Here's how the part is built. I have some questions about the finished solid (model axes, mm). A direction names the side the tool comes from. Round coordinates to 2 decimals unless told otherwise and drop trailing zeros. Order: outer loops, then holes, each group sorted by start corner. A loop starts at its lowest first (then second) coordinate and runs counter-clockwise, first axis right, second up. Notation, with made-up numbers: (78.5, 36.25) -> (130.5, 36.25) arc R27 ccw to (130.5, 69.25) -> close; hole circle Ø3 at (21.5, 54). An arc over 180 degrees is marked (long way). Answer in a Markdown table with one row per item.
```python
from build123d import *

# Parameters (mm, degrees)
F1_DEPTH  = 14
F3_W      = 7
F3_H      = 3.5
F4_DEPTH  = 16
F5_W      = 5
F5_H      = 0.4111507442
F5_H_2    = 17
F6_DEPTH  = 1.9
F8_R      = 0.99999
F10_DEPTH = 1.5
F11_W     = 2.5
F11_H     = 18.2
F12_DEPTH = 4.2
F13_W     = 2.5
F13_H     = 18.2
F14_DEPTH = 1.35
F15_W     = 3
F15_H     = 3
F16_DEPTH = 0.1
F17_DEPTH = 15
F18_R     = 5
F19_W     = 2.0917450339
F19_H     = 2.5
F20_DEPTH = 28.001
F19_W_2   = 2.772427164
F21_DEPTH = 28.001


# Not quite as in the source:
# - a fillet or chamfer is up to 0.001 mm smaller than in the source, because OpenCascade refuses the exact size
# - the program builds the solid bodies; features that only make, move or delete a surface that nothing else refers to are left out


with BuildPart() as f1:
    # F0 (on Front) → F1 (new body, symmetric)
    with BuildSketch(Plane.XZ):
        with BuildLine():
            Line((10, -6), (14, -6))
            Line((14, -6), (14, 6))
            Line((14, 6), (-14, 6))
            Line((-14, 6), (-14, -6))
            Line((-14, -6), (-10, -6))
            Line((-10, -6), (-4.7058823529, -3.1764705882))
            ThreePointArc((-4.7058823529, -3.1764705882), (0, -2), (4.7058823529, -3.1764705882))
            Line((4.7058823529, -3.1764705882), (10, -6))
        make_face()
        with BuildLine():
            Line((-10, -6), (10, -6))
            Line((10, -6), (4.7058823529, -3.1764705882))
            ThreePointArc((4.7058823529, -3.1764705882), (0, -2), (-4.7058823529, -3.1764705882))
            Line((-4.7058823529, -3.1764705882), (-10, -6))
        make_face()
    extrude(amount=F1_DEPTH, both=True)

    # F3 (on face) → F4 (cut)
    with BuildSketch(Plane.XZ.offset(14)):
        with Locations((0, 4.25)):
            Rectangle(F3_W, F3_H)
    extrude(amount=-F4_DEPTH, mode=Mode.SUBTRACT)

    # F5 (on face) → F6 (join)
    with BuildSketch(Plane.XY.offset(6)):
        with BuildLine():
            Line((2.5, -15), (-2.5, -15))
            Line((-2.5, -15), (-4, -15))
            ThreePointArc((-4, -15), (-5.4142135624, -15.5857864376), (-6, -17))
            Line((-6, -17), (-6, -18.5))
            ThreePointArc((-6, -18.5), (-5.267766953, -20.267766953), (-3.5, -21))
            Line((-3.5, -21), (3.5, -21))
            ThreePointArc((3.5, -21), (5.267766953, -20.267766953), (6, -18.5))
            Line((6, -18.5), (6, -17))
            ThreePointArc((6, -17), (5.4142135624, -15.5857864376), (4, -15))
            Line((4, -15), (2.5, -15))
        make_face()
        with Locations((0, 2.2055753721)):
            Rectangle(F5_W, F5_H)
        with Locations((0, -6.5)):
            Rectangle(F5_W, F5_H_2)
    extrude(amount=-F6_DEPTH)

    # F7: union 

    # F8 (radius 1 in the source; OpenCascade refuses exactly that, so slightly less here)
    f8_edges = [f1.edges().sort_by_distance(p)[0] for p in [
        (-3.5, -14, 4.25),
        (3.5, -14, 4.25),
        (2.5, 2, 5.05),
        (-2.5, 2, 5.05),
    ]]
    fillet(f8_edges, radius=F8_R)

    # F9 (on Right) → F10 (join, symmetric)
    with BuildSketch(Plane.YZ):
        Polygon((-6.6, 6), (-7.6, 7.5), (-9.1, 7.5), (-9.1, 6), align=None)
    extrude(amount=F10_DEPTH, both=True)

    # F11 (on face) → F12 (join)
    with BuildSketch(Plane.XY.offset(6)):
        with Locations((-9.25, 0)):
            Rectangle(F11_W, F11_H)
        with Locations((9.25, 0)):
            Rectangle(F11_W, F11_H)
    extrude(amount=F12_DEPTH)

    # F13 (on face) → F14 (join)
    with BuildSketch(Plane.XY.offset(10.2)):
        with Locations((-9.25, 0)):
            Rectangle(F13_W, F13_H)
        Polygon((-5.45, 9.1), (-8, 9.1), (-8, -9.1), (-5.2, -9.1), align=None)
        Polygon((5.45, 9.1), (5.2, -9.1), (10.5, -9.1), (10.5, 9.1), align=None)
    extrude(amount=-F14_DEPTH)

    # F15 (on face) → F16 (cut)
    with BuildSketch(Plane.XY.offset(6)):
        with Locations((0, 8.5)):
            Rectangle(F15_W, F15_H)
        Polygon((2.5, 7), (1.5, 7), (-1.5, 7), (-2.5, 7), (0, 4), align=None)
    extrude(amount=-F16_DEPTH, mode=Mode.SUBTRACT)

    # F2 (on Right) → F17 (cut, symmetric)
    with BuildSketch(Plane.YZ):
        with BuildLine():
            Line((-10, -6), (10, -6))
            Line((10, -6), (4.7058823529, -3.1764705882))
            ThreePointArc((4.7058823529, -3.1764705882), (0, -2), (-4.7058823529, -3.1764705882))
            Line((-4.7058823529, -3.1764705882), (-10, -6))
        make_face()
    extrude(amount=F17_DEPTH, both=True, mode=Mode.SUBTRACT)

    # F18
    f18_edges = [f1.edges().sort_by_distance(p)[0] for p in [
        (0, -10, -6),
        (0, 10, -6),
    ]]
    fillet(f18_edges, radius=F18_R)

    # F19 (on face) → F20 (cut, through all)
    with BuildSketch(Plane.XZ.offset(14)):
        with Locations((-10.2958725169, 1.25)):
            Rectangle(F19_W, F19_H)
    extrude(amount=-F20_DEPTH, mode=Mode.SUBTRACT)

    # F19 (on face) → F21 (cut, through all)
    with BuildSketch(Plane.XZ.offset(14)):
        with Locations((-10.2958725169, 1.25)):
            Rectangle(F19_W, F19_H)
        with Locations((9.9555305205, 1.25)):
            Rectangle(F19_W_2, F19_H)
    extrude(amount=-F21_DEPTH, mode=Mode.SUBTRACT)


solid = f1.part
```
1. Suppose I cut it at A-A on y = -6. State how many separate pieces and enclosed holes the cut face has, then the cut area to 3 significant figures.
Numbers:
| item | result |
|---|---|
| separate pieces | 2 |
| enclosed holes | 2 |
| area | 278 mm2 |
2. Please list where these lines run through material, in increasing order: line 1 along X through (y, z) = (-5.5, 5.5); line 2 along X through (y, z) = (2.5, 7); line 3 along X through (y, z) = (-1, 2.75).
Numbers:
| item | result |
|---|---|
| line 1 | x = -14 to -3.5, -2.5 to 2.5, 3.5 to 14 |
| line 2 | x = -10.5 to -8, 8 to 10.5 |
| line 3 | x = -14 to -3.5, 3.5 to 14 |
3. Suppose I cut it at D-D on x = 11.75. Write out the boundary of the cut face in (y, z), then the cut area to 3 significant figures.
Numbers:
| item | result |
|---|---|
| outline | (-14, -6) -> (-11.25, -6) arc R5 ccw to (-8.9, -5.41) -> (-4.71, -3.18) arc R10 cw to (4.71, -3.18) -> (8.9, -5.41) arc R5 ccw to (11.25, -6) -> (14, -6) -> (14, 6) -> (-14, 6) -> close |
| area | 287 mm2 |
4. For faces 1 (the face through (0, 2, 3)), 2 (the face through (-10, 0, 0)), 3 (the face through (-9, 9.1, 9)), 4 (the face through (3, -15, 5)), which set-ups out of +Z, -Z, +X, -X, +Y, -Y let a thin tool reach every point of the face, with its end or its side?
Numbers:
| item | result |
|---|---|
| face 1 | -Y |
| face 2 | +Y, -Y |
| face 3 | +Z, +X, -X, +Y |
| face 4 | +Z, -Z, +X |
5. Suppose I cut it at C-C on z = -4.5. Write out the boundary of the cut face in (x, y).
Numbers:
| item | result |
|---|---|
| outline | (-14, -14) -> (14, -14) -> (14, -7.19) -> (-14, -7.19) -> close; (-14, 7.19) -> (14, 7.19) -> (14, 14) -> (-14, 14) -> close |
6. For pin 1 Ø5 at (y, z) = (-12.5, 8) entering from +X; pin 2 Ø1.3 at (x, z) = (-9, 7.5) entering from -Y; pin 3 Ø1.5 at (x, y) = (-3.5, 8.5) entering from -Z; pin 4 Ø8 at (x, z) = (-5, -3) entering from -Y, each with a flat end and sliding along its axis, tell me the tip position at first contact or that it passes through.
Numbers:
| item | result |
|---|---|
| pin 1 | stops at x = 14 |
| pin 2 | stops at y = -9.1 |
| pin 3 | stops at z = -5.58 |
| pin 4 | stops at y = -14 |
7. Suppose I cut it at B-B on x = 6.5. Write out the boundary of the cut face in (y, z).
Numbers:
| item | result |
|---|---|
| outline | (-14, -6) -> (-11.25, -6) arc R5 ccw to (-8.9, -5.41) -> (-4.71, -3.18) arc R10 cw to (4.71, -3.18) -> (8.9, -5.41) arc R5 ccw to (11.25, -6) -> (14, -6) -> (14, 6) -> (-14, 6) -> close; (-9.1, 8.85) -> (9.1, 8.85) -> (9.1, 10.2) -> (-9.1, 10.2) -> close |
8. We'd pull the mould along Z, two halves only. Please class faces 5 (the face through (-10, 0, 2.5)), 6 (the face through (10.5, 0, 8)), 7 (the face through (11.342, 0, 1)): released by +Z, released by -Z, zero draft, split by the parting line, or undercut.
Numbers:
| item | result |
|---|---|
| face 5 | undercut |
| face 6 | zero draft |
| face 7 | undercut |
